CAD build for the part. Positions are in the model's coordinates, mm. Face numbers are marked on the shaded views. A direction names the side the tool comes from. Coordinates: 2 decimals unless noted, no trailing zeros. Loops run counter-clockwise (first coordinate to the right, second up) from the corner with the lowest first, then second, coordinate; pieces in that order, holes last. Notation, with made-up numbers: (48, 10) - (60, 10) arc R12 ccw to (60, 19) - close; hole circle Ø11 at (-36, -19.75). An arc over 180 degrees is marked (long way). Put each result on its own line as item: value.
```python
from build123d import *

# Parameters (mm, degrees)
SKETCH1_W            = 26
SKETCH1_H            = 28
BOSS_EXTRUDE1_DEPTH  = 8.5
SKETCH2_R            = 5
BOSS_EXTRUDE2_DEPTH  = 2
M3_CLEARANCE_HOLE1_D = 3.2


with BuildPart() as part:
    # Sketch1 → Boss-Extrude1 (new body)
    with BuildSketch(Plane(origin=(0, 0, 0), x_dir=(1, 0, 0), z_dir=(0, 1, 0))):
        Rectangle(SKETCH1_W, SKETCH1_H)
    extrude(amount=BOSS_EXTRUDE1_DEPTH)

    # Sketch2 → Boss-Extrude2 (add)
    with BuildSketch(Plane(origin=(0, 8.5, 0), x_dir=(1, 0, 0), z_dir=(0, 1, 0))):
        with Locations((-13, 1)):
            Circle(SKETCH2_R)
        with Locations((13, 1)):
            Circle(SKETCH2_R)
    extrude(amount=-BOSS_EXTRUDE2_DEPTH)

    # M3 Clearance Hole1 (through all)
    with Locations(Plane(origin=(0, 8.5, 0), x_dir=(1, 0, 0), z_dir=(0, 1, 0))):
        with Locations((-15.5, 1), (15.5, 1)):
            Hole(M3_CLEARANCE_HOLE1_D / 2)


solid = part.part
```
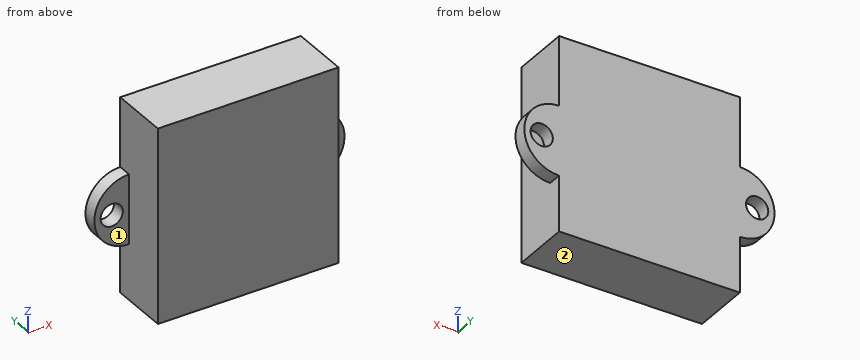
Q1. Wall check: L1, parallel to X at y = 7.5, z = -2.25; L2, parallel to X at y = 2, z = 4.75; L3, parallel to Y at x = 15, z = 1.75. Give the ranges that are in metal, low to high. Write a range as from..to.
Determined:
L1: -17.84..-16.5, -14.5..14.5, 16.5..17.84
L2: -13..13
L3: 6.5..8.5
Q2. Slice it at C-C, the plane y = 5.5. Give the cut face in (x, z).
Determined:
outline: (-13, -14) - (13, -14) - (13, 14) - (-13, 14) - close
Q3. Slice it at A-A, the plane z = -1. Give the cut face in (x, y), then the cut area to 3 significant figures.
Determined:
outline: (-18, 6.5) - (-17.1, 6.5) - (-17.1, 8.5) - (-18, 8.5) - close; (-13.9, 6.5) - (-13, 6.5) - (-13, 0) - (13, 0) - (13, 6.5) - (13.9, 6.5) - (13.9, 8.5) - (-13.9, 8.5) - close; (17.1, 6.5) - (18, 6.5) - (18, 8.5) - (17.1, 8.5) - close
area: 228 mm2
Q4. Slice it at D-D, the plane z = -8. Give the cut face in (x, y), then the cut area to 3 significant figures.
Determined:
outline: (-13, 0) - (13, 0) - (13, 8.5) - (-13, 8.5) - close
area: 221 mm2
Q5. Pin check, flat tips, straight feed: pin 1 Ø5 at (y, z) = (1, 6.5) entering from +X; pin 2 Ø4 at (y, z) = (5, -3) entering from +X; pin 3 Ø4 at (y, z) = (7.5, 10.5) entering from -X. Stop position of each tip, or through.
Determined:
pin 1: x = 13
pin 2: x = 17.95
pin 3: x = -13
Q6. Slice it at B-B, the plane x = 15.5. Give the cut face in (y, z).
Determined:
outline: (6.5, -5.33) - (8.5, -5.33) - (8.5, -2.6) - (6.5, -2.6) - close; (6.5, 0.6) - (8.5, 0.6) - (8.5, 3.33) - (6.5, 3.33) - close
Q7. Tool access for the marked faces 1 and 2: list every direction of +Z, -Z, +X, -X, +Y, -Y with a clear straight run to the whole face (end or side of a thin tool).
Determined:
face 1: +Z, -Z, -X, -Y
face 2: -Z, +X, -X, +Y, -Y
